Can you work these out from the model? Positions are in its coordinate system, mm. Round coordinates to 2 decimals unless told otherwise and drop trailing zeros. Order: outer loops, then holes, each group sorted by start corner. A loop starts at its lowest first (then second) coordinate and runs counter-clockwise, first axis right, second up. Notation, with made-up numbers: M -35,83.25 L -13,83.25 A31 ccw -13,107.25 Z; hole C 53,40 d10. An arc over 180 degrees is marked long. One line per question, with ' | ' between items.
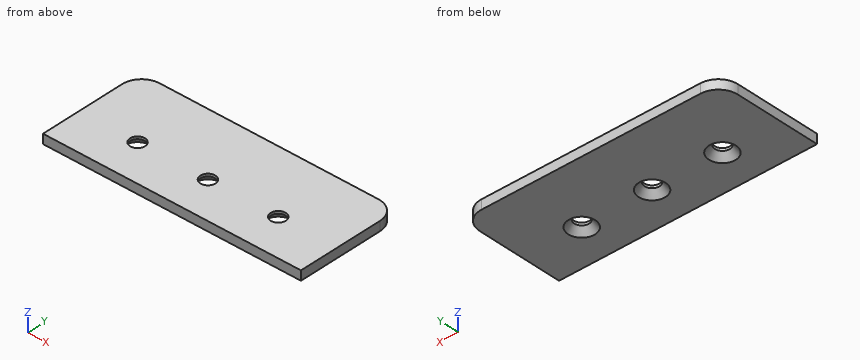
Autodesk Inventor part; units mm, degrees
ref_plane "YZ Plane" through (0, 0, 0) normal (1, 0, 0) x (0, 1, 0)
ref_plane "XZ Plane" through (0, 0, 0) normal (0, 1, 0) x (-1, 0, 0)
ref_plane "XY Plane" through (0, 0, 0) normal (0, 0, 1) x (1, 0, 0)
sketch "Sketch1" plane through (0, 0, 0) normal (0, 0, 1) x (1, 0, 0)
  line L0 (0, 20.574) -> (0, -3.429)
  line L1 (-29.337, 0) -> (29.337, 0)
  line L2 (20.955, 17.145) -> (-20.955, 17.145)
  line L3 (-20.955, 17.145) -> (-20.955, 0)
  line L4 (-20.955, 0) -> (20.955, 0)
  line L5 (20.955, 0) -> (20.955, 17.145)
  line L6 (20.955, 17.145) -> (-20.955, 0) construction
  line L7 (-20.955, 17.145) -> (20.955, 0) construction
  point P0 (0, 0)
  point P1 (0, 8.5725)
  point P2 (-11.43, 6.35)
  point P3 (0, 6.35)
  point P4 (11.43, 6.35)
  dimension "d0" = 41.91
  dimension "d1" = 17.145
  dimension "d2" = 11.43
  dimension "d3" = 11.43
  dimension "d4" = 6.35
extrude "Extrusion1" add sketch "Sketch1" along normal blind 1.524
fillet "Fillet1" radius 3.175 2 edges at (20.955, 17.145, 0.762) (-20.955, 17.145, 0.762)
hole "Hole1" at (-11.43, 6.35, 0) at (0, 6.35, 0) at (11.43, 6.35, 0) direction (0, 0, 1) diameter 2.4384 end through all countersink diameter 4.3688 countersink angle 82
properties material "DELRIN 100, BLACK (EXTRUDED)"
(1) If we section it at C-C on z = 0.6: Please give me the cut outline in (x, y) (3 decimals), plus the area to 3 significant figures.
Final values:
outline: M -20.955,0 L 20.955,0 L 20.955,13.97 A3.175 ccw 17.78,17.145 L -17.78,17.145 A3.175 ccw -20.955,13.97 Z; hole C -11.43,6.35 d3.326; hole C 0,6.35 d3.326; hole C 11.43,6.35 d3.326 | area: 688 mm^2
(2) Will this pin go through, and if not, where does the flat tip stop? pin 1 Ø3 at (x, y) = (0, 6.35) entering from -Z.
Final values:
pin 1: z = 0.79
(3) If we section it at A-A on x = -11.43: Please give me the cut outline in (y, z) (3 decimals).
Final values:
outline: M 0,0 L 4.166,0 L 5.131,1.11 L 5.131,1.524 L 0,1.524 Z; M 7.569,1.11 L 8.534,0 L 17.145,0 L 17.145,1.524 L 7.569,1.524 Z
(4) Please list where these lines run through material, in increasing order: probe 1 along X at (y, z) = (6.35, 1.35) (3 decimals); probe 2 along Y at (x, z) = (11.43, 1.4) (3 decimals); probe 3 along X at (y, z) = (5, 0.55) (3 decimals). Write a range as [from, to].
Final values:
probe 1: [-20.955, -12.649], [-10.211, -1.219], [1.219, 10.211], [12.649, 20.955] | probe 2: [0, 5.131], [7.569, 17.145] | probe 3: [-20.955, -12.474], [-10.386, -1.044], [1.044, 10.386], [12.474, 20.955]
(5) If we section it at B-B on y = 6.35: Please give me the cut outline in (x, z) (3 decimals), plus the area to 3 significant figures.
Final values:
outline: M -20.955,0 L -13.614,0 L -12.649,1.11 L -12.649,1.524 L -20.955,1.524 Z; M -10.211,1.11 L -9.246,0 L -2.184,0 L -1.219,1.11 L -1.219,1.524 L -10.211,1.524 Z; M 1.219,1.11 L 2.184,0 L 9.246,0 L 10.211,1.11 L 10.211,1.524 L 1.219,1.524 Z; M 12.649,1.11 L 13.614,0 L 20.955,0 L 20.955,1.524 L 12.649,1.524 Z | area: 49.5 mm^2
(6) If we section it at D-D on y = 16: Please give me the cut outline in (x, z).
Final values:
outline: M -20.22,0 L 20.22,0 L 20.22,1.52 L -20.22,1.52 Z
